```python
from build123d import *

# Parameters (mm, degrees)
SKETCH1_W           = 70
SKETCH1_H           = 25
BOSS_EXTRUDE1_DEPTH = 8
SKETCH4_W           = 20
SKETCH4_H           = 5
BOSS_EXTRUDE2_DEPTH = 50
CHAMFER1_SIZE       = 3
CUT_EXTRUDE5_DEPTH  = 92.761920207
FILLET13_R          = 5
FILLET14_R          = 2
FILLET15_R          = 1
SKETCH11_R          = 2.1
CUT_EXTRUDE6_DEPTH  = 10
FILLET18_R          = 3
FILLET20_R          = 1
SKETCH16_R          = 1.6
CUT_EXTRUDE11_DEPTH = 10
SKETCH17_R          = 4
CUT_EXTRUDE12_DEPTH = 4
SKETCH18_R          = 4
CUT_EXTRUDE13_DEPTH = 2


with BuildPart() as part:
    # Sketch1 → Boss-Extrude1 (new body)
    with BuildSketch(Plane.XY):
        Rectangle(SKETCH1_W, SKETCH1_H)
    extrude(amount=BOSS_EXTRUDE1_DEPTH)

    # Sketch4 → Boss-Extrude2 (add)
    with BuildSketch(Plane.XY.offset(8)):
        with Locations((-25, -10)):
            Rectangle(SKETCH4_W, SKETCH4_H)
    boss_extrude2 = extrude(amount=BOSS_EXTRUDE2_DEPTH)

    # Mirror1: Boss-Extrude2 across plane
    add(boss_extrude2.mirror(Plane.ZY))

    # Chamfer1
    chamfer1_edges = [part.edges().sort_by_distance(p)[0] for p in [
        (-35, 12.5, 4),
        (35, 12.5, 4),
    ]]
    chamfer(chamfer1_edges, length=CHAMFER1_SIZE)

    # Sketch10 → Cut-Extrude5 (cut, through all)
    with BuildSketch(Plane.ZY.offset(35)):
        Polygon((8, 11.3), (6, -5.5), (8, -5.5), align=None)
    extrude(amount=-CUT_EXTRUDE5_DEPTH, mode=Mode.SUBTRACT)

    # Fillet13
    fillet13_edges = [part.edges().sort_by_distance(p)[0] for p in [
        (-15, -10, 8),
        (15, -10, 8),
    ]]
    fillet(fillet13_edges, radius=FILLET13_R)

    # Fillet14
    fillet14_edges = [part.edges().sort_by_distance(p)[0] for p in [
        (22.5, -7.5, 8),
        (-22.5, -7.5, 8),
    ]]
    fillet(fillet14_edges, radius=FILLET14_R - 0.0001)  # a hair under: the kernel refuses the full size

    # Fillet15
    fillet15_edges = [part.edges().sort_by_distance(p)[0] for p in [
        (0, 12.5, 0),
        (0, -12.5, 0),
    ]]
    fillet(fillet15_edges, radius=FILLET15_R)

    # Sketch11 → Cut-Extrude6 (cut)
    with BuildSketch(Plane(origin=(0, -7.5, 0), x_dir=(1, 0, 0), z_dir=(0, 1, 0))):
        with Locations(Location((-25, -46, 0), (0, 0, 270))):
            Circle(SKETCH11_R)
        with Locations(Location((25, -46, 0), (0, 0, 270))):
            Circle(SKETCH11_R)
    extrude(amount=-CUT_EXTRUDE6_DEPTH, mode=Mode.SUBTRACT)

    # Fillet18
    fillet18_edges = [part.edges().sort_by_distance(p)[0] for p in [
        (-35, -10, 58),
        (-15, -10, 58),
        (35, -10, 58),
        (15, -10, 58),
    ]]
    fillet(fillet18_edges, radius=FILLET18_R)

    # Fillet20
    fillet20_edges = [part.edges().sort_by_distance(p)[0] for p in [
        (0, -5.5, 6),
    ]]
    fillet(fillet20_edges, radius=FILLET20_R)

    # Sketch16 → Cut-Extrude11 (cut)
    with BuildSketch(Plane(origin=(0, 0, 8), x_dir=(-1, 0, 0), z_dir=(0, 0, -1))):
        with Locations(Location((-22.5, 5, 0), (0, 0, 180))):
            Circle(SKETCH16_R)
        with Locations(Location((22.5, 5, 0), (0, 0, 180))):
            Circle(SKETCH16_R)
    extrude(amount=CUT_EXTRUDE11_DEPTH, mode=Mode.SUBTRACT)

    # Sketch17 → Cut-Extrude12 (cut)
    with BuildSketch(Plane(origin=(0, 0, 8), x_dir=(-1, 0, 0), z_dir=(0, 0, -1))):
        with Locations(Location((-22.5, 5, 0), (0, 0, 90))):
            Circle(SKETCH17_R)
        with Locations(Location((22.5, 5, 0), (0, 0, 90))):
            Circle(SKETCH17_R)
    extrude(amount=CUT_EXTRUDE12_DEPTH, mode=Mode.SUBTRACT)

    # Sketch18 → Cut-Extrude13 (cut)
    with BuildSketch(Plane(origin=(0, -7.5, 0), x_dir=(1, 0, 0), z_dir=(0, 1, 0))):
        with Locations(Location((-25, -46, 0), (0, 0, 270))):
            Circle(SKETCH18_R)
        with Locations(Location((25, -46, 0), (0, 0, 270))):
            Circle(SKETCH18_R)
    extrude(amount=-CUT_EXTRUDE13_DEPTH, mode=Mode.SUBTRACT)


solid = part.part
```
The model under review builds one solid part; all positions refer to its coordinate system, in mm. A direction names the side the tool comes from. Give positions to 0.01 mm unless a question says otherwise; leave off trailing zeros. Write each loop counter-clockwise with the first axis right and the second up, starting at its lowest first coordinate (ties: lowest second). Pieces come first, ordered by that corner, then holes. Notation, with made-up numbers: M -23.5,-1.75 L 7.5,-1.75 A10 ccw 7.5,17.25 Z; hole C 67.25,77 d1. An arc over 180 degrees is marked long. Write item = value, one per line. Start each with the question number.
Q1. We need section B-B (z = 36). State the section outline as (x, y) points, plus the area to 3 significant figures.
Q2. Clearance check with flat-ended pins moving along their axes: pin 1 (5 mm diameter, centred on x = 25, z = 46, fed in from +Y); pin 2 (10.5 mm diameter, centred on x = -22.5, y = 5, fed in from +Z) (3 decimals); pin 3 (23 mm diameter, centred on x = 23, z = 22.5, fed in from +Y); pin 4 (6 mm diameter, centred on x = -14.5, z = 24.5, fed in from -Y). State where each tip first meets the part, or that it passes through.
Q3. We need section A-A (z = 46). State the section outline as (x, y) points, plus the area to 3 significant figures.
Q4. For line 1 (X direction, y = 5, z = 5); line 2 (X direction, y = -8.7, z = 46); line 3 (Y direction, x = 22.5, z = 1.9), list the stretches that pass through material, from the lowest coordinate up.
Q5. Machinability: for faces 4 (the face through (-25, -7.5, 34)), 5 (the face through (28.966, -8.486, 45.479)), 6 (the face through (0, -9, 8)), 7 (the face through (-22, 7, 4)), which of the approach directions +Z, -Z, +X, -X, +Y, -Y give a long, thin tool a straight path to every point of the face, cutting with its end or side? Answer none if there is none.
Q6. We need section D-D (x = 3). State the section outline as (y, z) points, plus the area to 3 significant figures.
Q7. Mouldability with a two-part tool opening along X and no side actions: class faces 1 (the face through (-34.14, -9.96, 57.1)), 2 (the face through (34.14, -9.96, 57.1)), 3 (the face through (26.77, -10.98, 47.13)) as released by +X, released by -X, zero draft, split by the parting line, or undercut.
Result set:
q1.outline = M -35,-12.5 L -15,-12.5 L -15,-7.5 L -35,-7.5 Z; M 15,-12.5 L 35,-12.5 L 35,-7.5 L 15,-7.5 Z
q1.area = 200 mm2
q2.pin_1 = -9.5
q2.pin_2 = 7.875
q2.pin_3 = -7.5
q2.pin_4 = -12.5
q3.outline = M -35,-12.5 L -27.1,-12.5 L -27.1,-9.5 L -29,-9.5 L -29,-7.5 L -35,-7.5 Z; M -22.9,-12.5 L -15,-12.5 L -15,-7.5 L -21,-7.5 L -21,-9.5 L -22.9,-9.5 Z; M 15,-12.5 L 22.9,-12.5 L 22.9,-9.5 L 21,-9.5 L 21,-7.5 L 15,-7.5 Z; M 27.1,-12.5 L 35,-12.5 L 35,-7.5 L 29,-7.5 L 29,-9.5 L 27.1,-9.5 Z
q3.area = 143 mm2
q4.line_1 = -35 to -26.5, -18.5 to 18.5, 26.5 to 35
q4.line_2 = -35 to -29, -21 to -15, 15 to 21, 29 to 35
q4.line_3 = -12.5 to 3.4, 6.6 to 12.5
q5.face_4 = +Z, +X, -X, +Y
q5.face_5 = +Y
q5.face_6 = +Z, +Y, -Y
q5.face_7 = +Z
q6.outline = M -12.5,1 A1 ccw -11.5,0 L 11.5,0 A1 ccw 12.5,1 L 12.5,8 L 11.3,8 L -4.38,6.13 A1 cw -5.5,7.13 L -5.5,8 L -12.5,8 Z
q6.area = 183 mm2
q7.face_1 = released by -X
q7.face_2 = released by +X
q7.face_3 = undercut
